Geometry check sheet. Reference: the model listing, model coordinates, mm. Face numbers are marked on the shaded views. A direction names the side the tool comes from. Round coordinates to 2 decimals unless told otherwise and drop trailing zeros. Loops run counter-clockwise (first coordinate to the right, second up) from the corner with the lowest first, then second, coordinate; pieces in that order, holes last. Notation, with made-up numbers: (75, 42.5) -> (125, 42.5) arc R24 ccw to (125, 78.5) -> close; hole circle Ø9 at (13.25, 49.25). An arc over 180 degrees is marked (long way). Use one line per item in the form item = value.
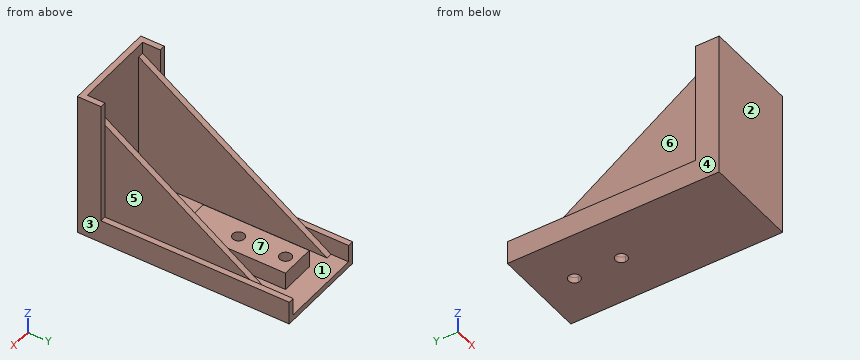
from build123d import *

# Parameters (mm, degrees)
SKETCH1_W               = 20
SKETCH1_H               = 31.25
BOSS_EXTRUDE1_DEPTH     = 2.5
CUT_EXTRUDE1_DEPTH      = 3.75
BOSS_EXTRUDE2_DEPTH     = 40
SKETCH4_W               = 1.25
SKETCH4_H               = 27.5
BOSS_EXTRUDE3_DEPTH     = 40
CUT_EXTRUDE5_DEPTH      = 16.25
CUT_EXTRUDE5_DEPTH_BACK = 1.25
SKETCH10_R              = 1.25
CUT_EXTRUDE6_DEPTH      = 45.75
CUT_EXTRUDE6_DEPTH_BACK = 2.25
SKETCH11_W              = 7.5
SKETCH11_H              = 22.5
BOSS_EXTRUDE4_DEPTH     = 3.75
SKETCH12_R              = 1.25
CUT_EXTRUDE7_DEPTH      = 13.75


with BuildPart() as part:
    # Sketch1 → Boss-Extrude1 (new body, symmetric)
    with BuildSketch(Plane(origin=(0, 0, 0), x_dir=(1, 0, 0), z_dir=(0, 1, 0))):
        with Locations((0, 1.875)):
            Rectangle(SKETCH1_W, SKETCH1_H)
    extrude(amount=BOSS_EXTRUDE1_DEPTH, both=True)

    # Sketch2 → Cut-Extrude1 (cut)
    with BuildSketch(Plane(origin=(0, 2.5, 0), x_dir=(1, 0, 0), z_dir=(0, 1, 0))):
        Polygon((-8.75, -12.5), (-8.75, -13.75), (8.75, -13.75), (8.75, -12.5), (8.75, 16.25), (-8.75, 16.25), align=None)
    extrude(amount=-CUT_EXTRUDE1_DEPTH, mode=Mode.SUBTRACT)

    # Sketch3 → Boss-Extrude2 (add)
    with BuildSketch(Plane(origin=(0, 2.5, 0), x_dir=(1, 0, 0), z_dir=(0, 1, 0))):
        Polygon((-8.75, 16.25), (-8.736970705, 16.25), (8.75, 16.25), (8.75, 12.5), (10, 12.5), (10, 17.5), (-8.732627572, 17.5), (-10, 17.5), (-10, 12.5), (-8.75, 12.5), align=None)
    extrude(amount=BOSS_EXTRUDE2_DEPTH)

    # Sketch4 → Boss-Extrude3 (add)
    with BuildSketch(Plane(origin=(0, -1.25, 0), x_dir=(1, 0, 0), z_dir=(0, 1, 0))):
        with Locations((8.125, 2.5)):
            Rectangle(SKETCH4_W, SKETCH4_H)
        with Locations((-8.125, 2.5)):
            Rectangle(SKETCH4_W, SKETCH4_H)
    extrude(amount=BOSS_EXTRUDE3_DEPTH)

    # Sketch7 → Cut-Extrude5 (cut, two sides)
    with BuildSketch(Plane.ZY.offset(-7.5)) as cut_extrude5_sk:
        Polygon((-16.25, 38.75), (11.25, 38.75), (11.25, -1.25), align=None)
    extrude(amount=CUT_EXTRUDE5_DEPTH, mode=Mode.SUBTRACT)
    extrude(cut_extrude5_sk.sketch, amount=-CUT_EXTRUDE5_DEPTH_BACK, mode=Mode.SUBTRACT)

    # Sketch10 → Cut-Extrude6 (cut, two sides)
    with BuildSketch(Plane.XY.offset(-16.25)) as cut_extrude6_sk:
        with Locations((0, 35)):
            Circle(SKETCH10_R)
        with Locations((0, 25)):
            Circle(SKETCH10_R)
    extrude(amount=CUT_EXTRUDE6_DEPTH, mode=Mode.SUBTRACT)
    extrude(cut_extrude6_sk.sketch, amount=-CUT_EXTRUDE6_DEPTH_BACK, mode=Mode.SUBTRACT)

    # Sketch11 → Boss-Extrude4 (add)
    with BuildSketch(Plane.XY.offset(-16.25)):
        with Locations((0, 26.25)):
            Rectangle(SKETCH11_W, SKETCH11_H)
    extrude(amount=BOSS_EXTRUDE4_DEPTH)

    # Sketch12 → Cut-Extrude7 (cut)
    with BuildSketch(Plane(origin=(0, 0, -17.5), x_dir=(-1, 0, 0), z_dir=(0, 0, -1))):
        with Locations((0, 35)):
            Circle(SKETCH12_R)
        with Locations((0, 25)):
            Circle(SKETCH12_R)
    extrude(amount=-CUT_EXTRUDE7_DEPTH, mode=Mode.SUBTRACT)


solid = part.part
1. Section check D-D (x = 4.5). Record the boundary of the cut face in (y, z).
Return value:
outline = (-2.5, -17.5) -> (42.5, -17.5) -> (42.5, -16.25) -> (-1.25, -16.25) -> (-1.25, 13.75) -> (-2.5, 13.75) -> close
2. Section check C-C (y = 28). Record the boundary of the cut face in (x, z).
Return value:
outline = (-10, -17.5) -> (10, -17.5) -> (10, -12.5) -> (8.75, -12.5) -> (8.75, -8.86) -> (7.5, -8.86) -> (7.5, -16.25) -> (3.75, -16.25) -> (3.75, -12.5) -> (-3.75, -12.5) -> (-3.75, -16.25) -> (-7.5, -16.25) -> (-7.5, -8.86) -> (-8.75, -8.86) -> (-8.75, -12.5) -> (-10, -12.5) -> close
3. Tool access check on the marked faces 4, 5, 6 and 7. Record the directions out of +Z, -Z, +X, -X, +Y, -Y that give a thin tool (end or side, any length) a straight path to the whole face; none if there is none.
Return value:
face_4 = +Z, -Z, -X, +Y, -Y
face_5 = +Z, +X, +Y
face_6 = +Z, -X, +Y
face_7 = +Z, +Y
4. Section check B-B (z = -14). Record the boundary of the cut face in (x, y), then the cut area to 3 significant figures.
Return value:
outline = (-10, -2.5) -> (10, -2.5) -> (10, 42.5) -> (8.75, 42.5) -> (8.75, 35.48) -> (7.5, 35.48) -> (7.5, -1.25) -> (-7.5, -1.25) -> (-7.5, 35.48) -> (-8.75, 35.48) -> (-8.75, 42.5) -> (-10, 42.5) -> close; (-3.75, 15) -> (3.75, 15) -> (3.75, 37.5) -> (-3.75, 37.5) -> close; hole circle Ø2.5 at (0, 25); hole circle Ø2.5 at (0, 35)
area = 385 mm2
5. Material ranges on line 1 along X through (y, z) = (25, -13); line 2 along Y through (x, z) = (0, -14.25); line 3 along X through (y, z) = (21, -9), recorded low to high.
Return value:
line_1 = -10 to -7.5, -3.75 to -1.25, 1.25 to 3.75, 7.5 to 10
line_2 = -2.5 to -1.25, 15 to 23.75, 26.25 to 33.75, 36.25 to 37.5
line_3 = -8.75 to -7.5, 7.5 to 8.75
6. Gauge pin test, flat ends, axial feed: pin 1 (17 mm diameter, centred on y = 15.5, z = -1, fed in from -X); pin 2 (5 mm diameter, centred on x = 2, z = 4.5, fed in from +Y); pin 3 (0.6 mm diameter, centred on x = -9.5, y = 20, fed in from +Z); pin 4 (2 mm diameter, centred on x = 0, y = 25, fed in from +Z) (1 decimal). Record the tip position at first contact, or that the pin passes through.
Return value:
pin_1 = -8.75
pin_2 = -1.25
pin_3 = -12.5
pin_4 = through
7. Mould release check, pull along Y, two halves, no side actions. Record for the marked faces 1, 2 and 3: released by +Y, released by -Y, zero draft, split by the parting line, or undercut.
Return value:
face_1 = undercut
face_2 = released by -Y
face_3 = zero draft
8. Section check A-A (x = 0). Record the boundary of the cut face in (y, z).
Return value:
outline = (-2.5, -17.5) -> (23.75, -17.5) -> (23.75, -12.5) -> (15, -12.5) -> (15, -16.25) -> (-1.25, -16.25) -> (-1.25, 13.75) -> (-2.5, 13.75) -> close; (26.25, -17.5) -> (33.75, -17.5) -> (33.75, -12.5) -> (26.25, -12.5) -> close; (36.25, -17.5) -> (42.5, -17.5) -> (42.5, -16.25) -> (37.5, -16.25) -> (37.5, -12.5) -> (36.25, -12.5) -> close
